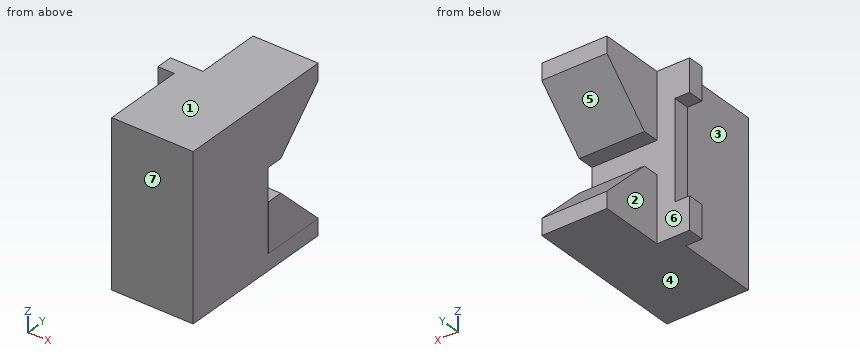
from build123d import *

# Parameters (mm, degrees)
SKETCH1_W            = 25
SKETCH1_H            = 50
BOSS_EXTRUDE1_DEPTH  = 25
SKETCH2_W            = 5
SKETCH2_H            = 10
BOSS_EXTRUDE2_DEPTH  = 5
SKETCH3_W            = 25
SKETCH3_H            = 50
BOSS_EXTRUDE3_DEPTH  = 5
SKETCH4_W            = 5
SKETCH4_H            = 10
BOSS_EXTRUDE5_DEPTH  = 5
SKETCH6_W            = 30.0479401
SKETCH6_H            = 5
BOSS_EXTRUDE6_DEPTH  = 0.5
SKETCH8_W            = 20
SKETCH8_H            = 5
BOSS_EXTRUDE7_DEPTH  = 20
SKETCH18_W           = 20
SKETCH18_H           = 15
BOSS_EXTRUDE9_DEPTH  = 20
CUT_EXTRUDE7_DEPTH   = 20
SKETCH15_W           = 20.034641196
SKETCH15_H           = 15
SKETCH15_W_2         = 20
SKETCH15_H_2         = 20
BOSS_EXTRUDE11_DEPTH = 20
CUT_EXTRUDE9_DEPTH   = 30


with BuildPart() as part:
    # Sketch1 → Boss-Extrude1 (new body)
    with BuildSketch(Plane(origin=(0, 0, 0), x_dir=(1, 0, 0), z_dir=(0, 1, 0))):
        with Locations((12.5, -25)):
            Rectangle(SKETCH1_W, SKETCH1_H)
    extrude(amount=BOSS_EXTRUDE1_DEPTH)



with BuildPart() as body_2:
    # Sketch2 → Boss-Extrude2 (new body)
    with BuildSketch(Plane(origin=(0, 25, 0), x_dir=(1, 0, 0), z_dir=(0, 1, 0))):
        with Locations((-2.5, -5)):
            Rectangle(SKETCH2_W, SKETCH2_H)
    extrude(amount=BOSS_EXTRUDE2_DEPTH)


with BuildPart() as part_1:
    add(part.part)

    add(body_2.part)  # Boss-Extrude3 merges body 2
    # Sketch3 → Boss-Extrude3 (add)
    with BuildSketch(Plane(origin=(0, 25, 0), x_dir=(1, 0, 0), z_dir=(0, 1, 0))):
        with Locations((12.5, -25)):
            Rectangle(SKETCH3_W, SKETCH3_H)
    extrude(amount=BOSS_EXTRUDE3_DEPTH)

    # Sketch4 → Boss-Extrude5 (add)
    with BuildSketch(Plane(origin=(0, 30, 0), x_dir=(1, 0, 0), z_dir=(0, 1, 0))):
        with Locations((-2.5, -45)):
            Rectangle(SKETCH4_W, SKETCH4_H)
    extrude(amount=-BOSS_EXTRUDE5_DEPTH)

    # Sketch6 → Boss-Extrude6 (add)
    with BuildSketch(Plane.ZY):
        with Locations((25.02397005, 27.5)):
            Rectangle(SKETCH6_W, SKETCH6_H)
    extrude(amount=BOSS_EXTRUDE6_DEPTH)

    # Sketch8 → Boss-Extrude7 (add)
    with BuildSketch(Plane(origin=(0, 30, 0), x_dir=(1, 0, 0), z_dir=(0, 1, 0))):
        with Locations((15, -2.5)):
            Rectangle(SKETCH8_W, SKETCH8_H)
    extrude(amount=BOSS_EXTRUDE7_DEPTH)

    # Sketch18 → Boss-Extrude9 (add)
    with BuildSketch(Plane(origin=(0, 30, 0), x_dir=(1, 0, 0), z_dir=(0, 1, 0))):
        with Locations((15, -42.5)):
            Rectangle(SKETCH18_W, SKETCH18_H)
    extrude(amount=BOSS_EXTRUDE9_DEPTH)

    # Sketch20 → Cut-Extrude7 (cut)
    with BuildSketch(Plane.ZY.offset(-5)):
        Polygon((45, 50), (35, 35), (35, 50), align=None)
    extrude(amount=-CUT_EXTRUDE7_DEPTH, mode=Mode.SUBTRACT)

    # Sketch15 → Boss-Extrude11 (add)
    with BuildSketch(Plane(origin=(0, 30, 0), x_dir=(1, 0, 0), z_dir=(0, 1, 0))):
        with Locations((15.017320598, -12.5)):
            Rectangle(SKETCH15_W, SKETCH15_H)
        with Locations((15, -40)):
            Rectangle(SKETCH15_W_2, SKETCH15_H_2)
    extrude(amount=BOSS_EXTRUDE11_DEPTH)

    # Sketch21 → Cut-Extrude9 (cut)
    with BuildSketch(Plane.ZY.offset(-5)):
        Polygon((5, 50), (20, 50), (20, 35), align=None)
        Polygon((45, 50), (30, 35), (30, 50), align=None)
    extrude(amount=-CUT_EXTRUDE9_DEPTH, mode=Mode.SUBTRACT)


solid = part_1.part
The model under review builds one solid part; all positions refer to its coordinate system, in mm. Face numbers are marked on the shaded views. A direction names the side the tool comes from. Round coordinates to 2 decimals unless told otherwise and drop trailing zeros. Write each loop counter-clockwise with the first axis right and the second up, starting at its lowest first coordinate (ties: lowest second). Pieces come first, ordered by that corner, then holes. Notation, with made-up numbers: M -10,89 L 21,89 A29 cw 21,110 Z; hole C -27.75,4 d9. An arc over 180 degrees is marked long. Use a Markdown table: item, result. Add a question column.
Q1. Machinability: for the marked faces 1, 2 and 3, which of the approach directions +Z, -Z, +X, -X, +Y, -Y give a long, thin tool a straight path to every point of the face, cutting with its end or side? Answer none if there is none.
Q2. The part is to be moulded in two halves that separate along Z. For the marked faces 4, 5, 6 and 7, say which applies: pulls with the +Z half, pulls with the -Z half, needs draft (parallel to the pull), parting line crosses it, or undercut.
Q3. We need section D-D, the plane x = 15. State the section outline as (y, z) points.
Q4. Insertion check: pin 1 (2 mm diameter, centred on y = 41, z = 6.5, fed in from -X); pin 2 (20 mm diameter, centred on y = 14.5, z = 19.5, fed in from -X); pin 3 (9 mm diameter, centred on x = 7.5, z = 19, fed in from +Y); pin 4 (2.5 mm diameter, centred on x = 10, y = 32, fed in from -Z). Each pin has a flat end and moves straight along its axis. Give the tip position at first contact, or say it passes through.
Q5. We need section B-B, the plane z = 33.5. State the section outline as (x, y) points.
Q6. To check wall thickness, follow line 1 (Z direction, x = 12, y = 33); line 2 (X direction, y = 46, z = 42); line 3 (X direction, y = 23.5, z = 15.5). State the ranges of each line that lie inside material, in increasing order.
Q7. We need section C-C, the plane x = -2. State the section outline as (y, z) points, plus the area to 3 significant figures.
Findings below:
| question | item | result |
|---|---|---|
| 1 | face 1 | +Z, +X, -X, +Y, -Y |
| 1 | face 2 | +Z, -Z, -X, +Y |
| 1 | face 3 | +Z, -Z, -X, -Y |
| 2 | face 4 | pulls with the -Z half |
| 2 | face 5 | undercut |
| 2 | face 6 | undercut |
| 2 | face 7 | needs draft |
| 3 | outline | M 0,0 L 50,0 L 50,5 L 35,20 L 30,20 L 30,30 L 35,30 L 50,45 L 50,50 L 0,50 Z |
| 4 | pin 1 | stops at x = 5 |
| 4 | pin 2 | stops at x = 0 |
| 4 | pin 3 | stops at y = 40.5 |
| 4 | pin 4 | stops at z = 0 |
| 5 | outline | M -0.5,25 L 0,25 L 0,0 L 25,0 L 25,38.5 L 5,38.5 L 5,30 L -0.5,30 Z |
| 6 | line 1 | z = 0 to 20, 30 to 50 |
| 6 | line 2 | x = 5 to 25 |
| 6 | line 3 | x = 0 to 25 |
| 7 | outline | M 25,0 L 30,0 L 30,10 L 25,10 Z; M 25,40 L 30,40 L 30,50 L 25,50 Z |
| 7 | area | 100 mm² |
